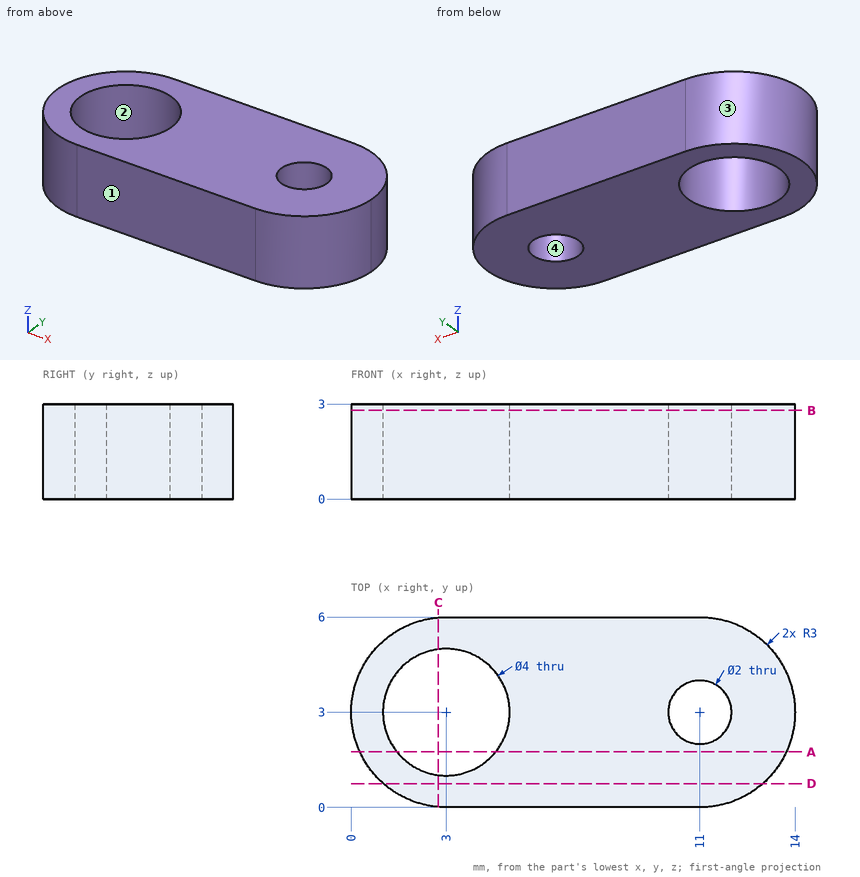
Input: dimensioned drawing with shaded views. Units: mm. Origin: part minimum x, y, z. Round coordinates to 2 decimals unless told otherwise and drop trailing zeros. Write each loop counter-clockwise with the first axis right and the second up, starting at its lowest first coordinate (ties: lowest second). Pieces come first, ordered by that corner, then holes. Notation, with made-up numbers: (-28.75, 25.5) -> (20.25, 25.5) arc R20 cw to (20.25, 62.5) -> close; hole circle Ø5 at (-27, -19). An arc over 180 degrees is marked (long way). Use CSV: the item, a comma, the result in double quotes. Start each with the question number.
Q1. Pull-direction query (X, two-part tool) for the marked faces 1, 2, 3 and 4; classes: pulls with the +X half, pulls with the -X half, needs draft (parallel to the pull), parting line crosses it, or undercut.
Q2. Line query: L1, parallel to Y at x = 3, z = 1.6; L2, parallel to Y at x = 11, z = 1.8; L3, parallel to X at y = 2.25, z = 1.45. Output: solid intervals per line, ascending.
Q3. First-contact query: pin 1 Ø1.5 at (y, z) = (4.5, 0.5) entering from +X. Flat tip, straight axial feed; report the tip coordinate or a pass-through.
Q4. Section B-B (z = 2.8). Return loops of the section in (x, y), plus the area to 3 significant figures.
Q5. Section A-A (y = 1.75). Return loops of the section in (x, z).
Q6. Section C-C (x = 2.75). Return loops of the section in (y, z).
Q7. Section D-D (y = 0.75). Return loops of the section in (x, z).
Result sheet:
1,face 1,"needs draft"
1,face 2,"undercut"
1,face 3,"pulls with the -X half"
1,face 4,"undercut"
2,L1,"0 to 1, 5 to 6"
2,L2,"0 to 2, 4 to 6"
2,L3,"0.1 to 1.15, 4.85 to 10.34, 11.66 to 13.9"
3,pin 1,"x = 13.9"
4,outline,"(3, 0) -> (11, 0) arc R3 ccw to (11, 6) -> (3, 6) arc R3 ccw to start; hole circle Ø4 at (3, 3); hole circle Ø2 at (11, 3)"
4,area,"60.6 mm²"
5,outline,"(0.27, 0) -> (1.44, 0) -> (1.44, 3) -> (0.27, 3) -> close; (4.56, 0) -> (13.73, 0) -> (13.73, 3) -> (4.56, 3) -> close"
6,outline,"(0.01, 0) -> (1.02, 0) -> (1.02, 3) -> (0.01, 3) -> close; (4.98, 0) -> (5.99, 0) -> (5.99, 3) -> (4.98, 3) -> close"
7,outline,"(1.02, 0) -> (12.98, 0) -> (12.98, 3) -> (1.02, 3) -> close"
